Part model, mm, in its own coordinate system. Face numbers are marked on the shaded views. A direction names the side the tool comes from. Give positions to 0.01 mm unless a question says otherwise; leave off trailing zeros. Write each loop counter-clockwise with the first axis right and the second up, starting at its lowest first coordinate (ties: lowest second). Pieces come first, ordered by that corner, then holes. Notation, with made-up numbers: (-11.75, 44) - (10.25, 44) arc R15 ccw to (10.25, 64) - close; hole circle Ø3 at (82, -38.75). An arc over 180 degrees is marked (long way). Answer as a JSON object with one key per item and string values. Group by question number.
```python
from build123d import *

# Parameters (mm, degrees)
F0_W     = 115
F0_H     = 160
F1_DEPTH = 10
F3_DEPTH = 10.001


# Not quite as in the source:
# - a pattern or mirror of a feature is missing from the dataset's text; its kind, count and spacing are read off the source's solid


with BuildPart() as f1:
    # F0 (on Top) → F1 (new body)
    with BuildSketch(Plane.XY):
        Rectangle(F0_W, F0_H)
        with BuildLine():
            Line((-22.5, -15), (-22.5, 15))
            ThreePointArc((-22.5, 15), (0, 37.5), (22.5, 15))
            Line((22.5, 15), (22.5, -15))
            ThreePointArc((22.5, -15), (0, -37.5), (-22.5, -15))
        make_face(mode=Mode.SUBTRACT)
    extrude(amount=F1_DEPTH)

    # F2 (on face) → F3 (cut, through all)
    with BuildSketch(Plane.XY.offset(10)):
        with BuildLine():
            ThreePointArc((-26, 15), (-30, 19), (-34, 15))
            Line((-34, 15), (-34, -15))
            ThreePointArc((-34, -15), (-30, -19), (-26, -15))
            Line((-26, -15), (-26, 0))
            Line((-26, 0), (-26, 15))
        make_face()
    f3 = extrude(amount=-F3_DEPTH, mode=Mode.SUBTRACT)

    # F3_copies: F3 across plane
    add(f3.mirror(Plane(origin=(0, 0, 0), x_dir=(0, 0, 1), z_dir=(1, 0, 0))), mode=Mode.SUBTRACT)


solid = f1.part
```
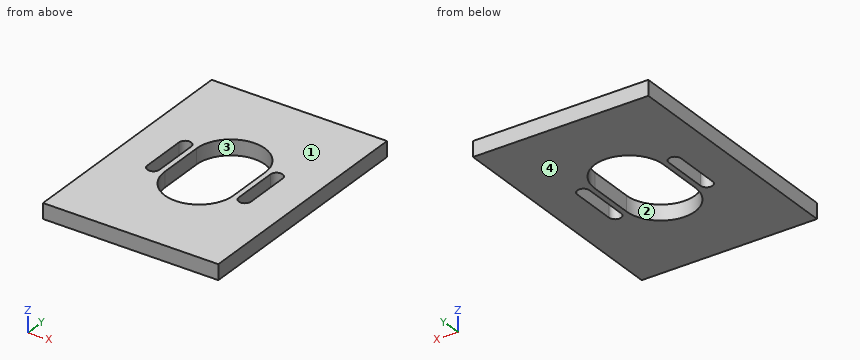
1) Band-saw the part on C-C (y = 5.5). List the corners of the cut face in (x, z), plus the area to 3 significant figures.
2) Mould opens along X. For the marked faces 3 and 4 say: pulls with the +X half, pulls with the -X half, needs draft (parallel to the pull), parting line crosses it, or undercut.
3) Probe line 1 (X direction, y = 8, z = 4.5); line 2 (Y direction, x = 8, z = 8.5); line 3 (Y direction, x = 3, z = 9.25). List the from-to ranges inside material, lowest first.
4) Band-saw the part on A-A (x = -13.5). List the corners of the cut face in (y, z), plus the area to 3 significant figures.
5) Band-saw the part on B-B (z = 2.5). List the corners of the cut face in (x, y).
6) Which spindle directions (+Z, -Z, +X, -X, +Y, -Y) get a long thin tool onto all of the face, cutting with end or side? Do the marked faces 1 and 2. Say none if no direction does.
7) Band-saw the part on D-D (x = 0). List the corners of the cut face in (y, z).
Verdict:
{
 "1": {"outline": "(-57.5, 0) - (-34, 0) - (-34, 10) - (-57.5, 10) - close; (-26, 0) - (-22.5, 0) - (-22.5, 10) - (-26, 10) - close; (22.5, 0) - (26, 0) - (26, 10) - (22.5, 10) - close; (34, 0) - (57.5, 0) - (57.5, 10) - (34, 10) - close", "area": "540 mm2"},
 "2": {"face 3": "undercut", "face 4": "needs draft"},
 "3": {"line 1": "-57.5 to -34, -26 to -22.5, 22.5 to 26, 34 to 57.5", "line 2": "-80 to -36.03, 36.03 to 80", "line 3": "-80 to -37.3, 37.3 to 80"},
 "4": {"outline": "(-80, 0) - (-33, 0) - (-33, 10) - (-80, 10) - close; (33, 0) - (80, 0) - (80, 10) - (33, 10) - close", "area": "940 mm2"},
 "5": {"outline": "(-57.5, -80) - (57.5, -80) - (57.5, 80) - (-57.5, 80) - close; hole (-34, -15) arc R4 ccw to (-26, -15) - (-26, 15) arc R4 ccw to (-34, 15) - close; hole (-22.5, -15) arc R22.5 ccw to (22.5, -15) - (22.5, 15) arc R22.5 ccw to (-22.5, 15) - close; hole (26, -15) arc R4 ccw to (34, -15) - (34, 15) arc R4 ccw to (26, 15) - close"},
 "6": {"face 1": "+Z, +X, -X, +Y, -Y", "face 2": "+Z, -Z"},
 "7": {"outline": "(-80, 0) - (-37.5, 0) - (-37.5, 10) - (-80, 10) - close; (37.5, 0) - (80, 0) - (80, 10) - (37.5, 10) - close"}
}
